```python
from build123d import *

# Parameters (mm, degrees)
BOSS_EXTRUDE1_DEPTH             = 18
BOSS_EXTRUDE2_REACH             = 40.419
BOSS_EXTRUDE2_DIRECTION_2_DEPTH = 21
SKETCH10_W                      = 24
SKETCH10_H                      = 36
BOSS_EXTRUDE4_DEPTH             = 2.3
CUT_EXTRUDE1_DEPTH              = 58.967577144
CUT_EXTRUDE1_DEPTH_BACK         = 58.967577144
SKETCH4_R                       = 2.6605
SKETCH4_3_R                     = 2.75
CUT_EXTRUDE2_DEPTH              = 3.2
CUT_EXTRUDE3_DEPTH              = 55.920305899
CUT_EXTRUDE3_DEPTH_BACK         = 55.920305899
SKETCH6_R                       = 2
SKETCH8_R                       = 2
CUT_EXTRUDE4_DEPTH              = 58.967577144
SKETCH8_3_R                     = 4.25
SKETCH8_3_R_2                   = 2
CUT_EXTRUDE5_DEPTH              = 8.8


with BuildPart() as part:
    # Sketch1 → Boss-Extrude1 (new, symmetric)
    with BuildSketch(Plane.XY):
        with BuildLine():
            Line((0, 0), (4, 0))
            Line((4, 0), (4, 19.5))
            ThreePointArc((4, 19.5), (3.646446609, 20.353553391), (4.5, 20))
            Line((4.5, 20), (24, 20))
            Line((24, 20), (24, 24))
            Line((24, 24), (0, 24))
            Line((0, 24), (0, 0))
        make_face()
    extrude(amount=BOSS_EXTRUDE1_DEPTH, both=True)

    # Boss-Extrude2: up to this face of the body (flat: up to its plane)
    boss_extrude2_end = Plane(part.part.faces().sort_by_distance((0, 12, 0))[0])
    # Sketch3 → Boss-Extrude2 (add, up to the picked face)
    with BuildSketch(Plane.ZY.offset(-24), mode=Mode.PRIVATE) as boss_extrude2_sk1:
        with BuildLine():
            ThreePointArc((8.919270833, 22.125269034), (6.25, 23.11319686), (3.580729167, 22.125269034))
            ThreePointArc((3.580729167, 22.125269034), (0, 20.8), (-3.580729167, 22.125269034))
            ThreePointArc((-3.580729167, 22.125269034), (-6.25, 23.11319686), (-8.919270833, 22.125269034))
            ThreePointArc((-8.919270833, 22.125269034), (-18, 26.3), (-8.919270833, 30.474730966))
            ThreePointArc((-8.919270833, 30.474730966), (-6.25, 29.48680314), (-3.580729167, 30.474730966))
            ThreePointArc((-3.580729167, 30.474730966), (0, 31.8), (3.580729167, 30.474730966))
            ThreePointArc((3.580729167, 30.474730966), (6.25, 29.48680314), (8.919270833, 30.474730966))
            ThreePointArc((8.919270833, 30.474730966), (18, 26.3), (8.919270833, 22.125269034))
        make_face()
    boss_extrude2_tool1 = split(extrude(boss_extrude2_sk1.sketch, amount=BOSS_EXTRUDE2_REACH, mode=Mode.PRIVATE), bisect_by=boss_extrude2_end, keep=Keep.BOTH, mode=Mode.PRIVATE)
    add(boss_extrude2_tool1.solids().sort_by(Axis((24, 26.3, 0), (-1, 0, 0)))[0])

    # Sketch3 → Boss-Extrude2 direction 2 (add)
    with BuildSketch(Plane.ZY.offset(-24)):
        with BuildLine():
            ThreePointArc((8.919270833, 22.125269034), (6.25, 23.11319686), (3.580729167, 22.125269034))
            ThreePointArc((3.580729167, 22.125269034), (0, 20.8), (-3.580729167, 22.125269034))
            ThreePointArc((-3.580729167, 22.125269034), (-6.25, 23.11319686), (-8.919270833, 22.125269034))
            ThreePointArc((-8.919270833, 22.125269034), (-18, 26.3), (-8.919270833, 30.474730966))
            ThreePointArc((-8.919270833, 30.474730966), (-6.25, 29.48680314), (-3.580729167, 30.474730966))
            ThreePointArc((-3.580729167, 30.474730966), (0, 31.8), (3.580729167, 30.474730966))
            ThreePointArc((3.580729167, 30.474730966), (6.25, 29.48680314), (8.919270833, 30.474730966))
            ThreePointArc((8.919270833, 30.474730966), (18, 26.3), (8.919270833, 22.125269034))
        make_face()
    extrude(amount=-BOSS_EXTRUDE2_DIRECTION_2_DEPTH)

    # Sketch10 → Boss-Extrude4 (add)
    with BuildSketch(Plane(origin=(0, 24, 0), x_dir=(1, 0, 0), z_dir=(0, 1, 0))):
        with Locations((12, 0)):
            Rectangle(SKETCH10_W, SKETCH10_H)
    extrude(amount=BOSS_EXTRUDE4_DEPTH)

    # Sketch4 → Cut-Extrude1 (cut, two sides: drawn at the far end of the back side and taken through both)
    with BuildSketch(Plane(origin=(45, 0, 0), x_dir=(0, 0, -1), z_dir=(1, 0, 0)).offset(-CUT_EXTRUDE1_DEPTH_BACK)):
        with Locations((-12.5, 26.3)):
            Circle(SKETCH4_R)
        with Locations((12.5, 26.3)):
            Circle(SKETCH4_R)
    extrude(amount=CUT_EXTRUDE1_DEPTH + CUT_EXTRUDE1_DEPTH_BACK, mode=Mode.SUBTRACT)

    # Sketch4<3> → Cut-Extrude2 (cut)
    with BuildSketch(Plane(origin=(45, 0, 0), x_dir=(0, 0, -1), z_dir=(1, 0, 0))):
        with Locations((0, 26.3)):
            Circle(SKETCH4_3_R)
    extrude(amount=-CUT_EXTRUDE2_DEPTH, mode=Mode.SUBTRACT)

    # Sketch6 → Cut-Extrude3 (cut, two sides: drawn at the far end of the back side and taken through both)
    with BuildSketch(Plane(origin=(4, 0, 0), x_dir=(0, 0, -1), z_dir=(1, 0, 0)).offset(-CUT_EXTRUDE3_DEPTH_BACK)):
        with Locations((-9, 10)):
            Circle(SKETCH6_R)
        with Locations((9, 10)):
            Circle(SKETCH6_R)
    extrude(amount=CUT_EXTRUDE3_DEPTH + CUT_EXTRUDE3_DEPTH_BACK, mode=Mode.SUBTRACT)

    # Sketch8 → Cut-Extrude4 (cut, through all)
    with BuildSketch(Plane(origin=(0, 31.8, 0), x_dir=(1, 0, 0), z_dir=(0, 1, 0))):
        with Locations(Location((14, 0, 0), (0, 0, 270))):
            Circle(SKETCH8_R)
    extrude(amount=-CUT_EXTRUDE4_DEPTH, mode=Mode.SUBTRACT)

    # Sketch8<3> → Cut-Extrude5 (cut)
    with BuildSketch(Plane(origin=(0, 31.8, 0), x_dir=(1, 0, 0), z_dir=(0, 1, 0))):
        with Locations(Location((14, 0, 0), (0, 0, 270))):
            Circle(SKETCH8_3_R)
        with Locations(Location((14, 0, 0), (0, 0, 270))):
            Circle(SKETCH8_3_R_2, mode=Mode.SUBTRACT)
    extrude(amount=-CUT_EXTRUDE5_DEPTH, mode=Mode.SUBTRACT)


solid = part.part
```
The listing builds one solid part. Answer for the finished solid, in the listing's coordinates (mm). A direction names the side the tool comes from. Give positions to 0.01 mm unless a question says otherwise; leave off trailing zeros. Order: outer loops, then holes, each group sorted by start corner. A loop starts at its lowest first (then second) coordinate and runs counter-clockwise, first axis right, second up.
Item 1: Find the intervals of material crossed by probe 1 along Z at (x, y) = (33.5, 26); probe 2 along Z at (x, y) = (19, 25); probe 3 along Y at (x, z) = (15.5, 12.5), in increasing order.
From the geometry:
probe 1: z = -17.99 to -15.14, -9.86 to 9.86, 15.14 to 17.99
probe 2: z = -18 to -14.82, -10.18 to 10.18, 14.82 to 18
probe 3: y = 20 to 23.64, 28.96 to 31.8
Item 2: For a pull along Z with two mould halves and no side action, classify faces 1 (the face through (4, 10, 0)), 2 (the face through (2, 12, 9)) as pulls with the +Z half, pulls with the -Z half, needs draft (parallel to the pull), parting line crosses it, or undercut.
From the geometry:
face 1: needs draft
face 2: undercut
Item 3: Which of the six approach directions +Z, -Z, +X, -X, +Y, -Y give full straight-line access (tool end or side, diameter ignored) to faces 3 (the face through (24, 20.6, 1.4)), 4 (the face through (22.185, 26.417, -9.842)), 5 (the face through (27.18, 29.12, 17.22)), 6 (the face through (16.3, 20, 0.3))?
From the geometry:
face 3: +X, -Y
face 4: +X, -X
face 5: +X
face 6: +Z, -Z, +X, -Y
Item 4: The part is cut by section C-C, the plane z = 0. Give the vertices of the cut face in (x, y).
From the geometry:
outline: (0, 0) - (4, 0) - (4, 19.5) arc R0.5 cw (long way) to (4.5, 20) - (12, 20) - (12, 23) - (9.75, 23) - (9.75, 31.8) - (0, 31.8) - close; (16, 20) - (24, 20) - (24, 20.8) - (45, 20.8) - (45, 23.55) - (41.8, 23.55) - (41.8, 29.05) - (45, 29.05) - (45, 31.8) - (18.25, 31.8) - (18.25, 23) - (16, 23) - close
Item 5: The part is cut by section D-D, the plane x = 34. Give the vertices of the cut face in (y, z), and give its area (3 significant figures).
From the geometry:
outline: (22.13, -8.92) arc R5.5 ccw (long way) to (30.47, -8.92) arc R4.1 cw to (30.47, -3.58) arc R5.5 ccw to (30.47, 3.58) arc R4.1 cw to (30.47, 8.92) arc R5.5 ccw (long way) to (22.13, 8.92) arc R4.1 cw to (22.13, 3.58) arc R5.5 ccw to (22.13, -3.58) arc R4.1 cw to start; hole circle Ø5.32 at (26.3, -12.5); hole circle Ø5.32 at (26.3, 12.5)
area: 271 mm2
Item 6: The part is cut by section A-A, the plane z = -12.5. Give the vertices of the cut face in (x, y).
From the geometry:
outline: (0, 0) - (4, 0) - (4, 19.5) arc R0.5 cw (long way) to (4.5, 20) - (24, 20) - (24, 20.8) - (45, 20.8) - (45, 23.64) - (0, 23.64) - close; (0, 28.96) - (45, 28.96) - (45, 31.8) - (0, 31.8) - close
Item 7: The part is cut by section B-B, the plane x = 20. Give the vertices of the cut face in (y, z), and give its area (3 significant figures).
From the geometry:
outline: (20, -18) - (26.3, -18) arc R5.5 ccw to (30.47, -8.92) arc R4.1 cw to (30.47, -3.58) arc R5.5 ccw to (30.47, 3.58) arc R4.1 cw to (30.47, 8.92) arc R5.5 ccw to (26.3, 18) - (20, 18) - close; hole circle Ø5.32 at (26.3, -12.5); hole circle Ø5.32 at (26.3, 12.5)
area: 340 mm2
Item 8: Given pin 1 Ø1.6 at (y, z) = (26, -0.5) entering from +X; pin 2 Ø6 at (x, z) = (15, 4) entering from -Y; pin 3 Ø7 at (x, z) = (14, 0.5) entering from +Y, each flat-ended and moving along its own axis, determine where each tip first touches the part or whether it passes through.
From the geometry:
pin 1: stops at x = 41.8
pin 2: stops at y = 20
pin 3: stops at y = 23
